Autodesk Inventor part; units mm, degrees
ref_plane "YZ Plane" through (0, 0, 0) normal (1, 0, 0) x (0, 1, 0)
ref_plane "XZ Plane" through (0, 0, 0) normal (0, 1, 0) x (-1, 0, 0)
ref_plane "XY Plane" through (0, 0, 0) normal (0, 0, 1) x (1, 0, 0)
sketch "Skizze1" plane through (0, 0, 0) normal (0, 1, 0) x (-1, 0, 0)
  line L0 (144.9597, 31.6532) -> (-5.0403, 31.6532)
  line L1 (-5.0403, 31.6532) -> (-5.0403, -118.3468)
  line L2 (-5.0403, -118.3468) -> (144.9597, -118.3468)
  line L3 (144.9597, -118.3468) -> (144.9597, 31.6532)
  line L4 (144.9597, 31.6532) -> (-5.0403, -118.3468) construction
  line L5 (-5.0403, 31.6532) -> (144.9597, -118.3468) construction
  point P0 (0, 0)
  point P1 (69.9597, -43.3468)
  dimension "d0" = 150
  dimension "d1" = 150
extrude "Extrusion1" add sketch "Skizze1" along normal blind 5
sketch "Skizze2" plane through (0, 5, 0) normal (0, 1, 0) x (1, 0, 0)
  circle A0 centre (-134.9597, -21.6532) radius 2.5
  circle A1 centre (-134.9597, 108.3468) radius 2.5
  circle A2 centre (-4.9597, -21.6532) radius 2.5
  circle A3 centre (-4.9597, 108.3468) radius 2.5
  line L0 (-144.9597, 118.3468) -> (-144.9597, -31.6532)
  line L1 (-144.9597, -31.6532) -> (5.0403, -31.6532)
  line L2 (5.0403, 118.3468) -> (-144.9597, 118.3468)
  line L3 (5.0403, -31.6532) -> (5.0403, 118.3468)
  point P0 (0, 0)
  dimension "d4" = 5
  dimension "d5" = 5
  dimension "d6" = 5
  dimension "d7" = 5
  dimension "d8" = 10
  dimension "d9" = 10
  dimension "d15" = 10
  dimension "d16" = 10
  dimension "d17" = 10
  dimension "d18" = 10
  dimension "d19" = 10
  dimension "d20" = 10
hole "Bohrung1" at (-134.9597, 5, 21.6532) at (-134.9597, 5, -108.3468) at (-4.9597, 5, -108.3468) at (-4.9597, 5, 21.6532) direction (0, -1, 0) diameter 4.978 depth 19.05 tip angle 118
sketch "Skizze3" plane through (0, 5, 0) normal (0, 1, 0) x (1, 0, 0)
  line L0 (-144.9597, 118.3468) -> (-144.9597, -31.6532)
  line L1 (-144.9597, 18.3468) -> (-124.9597, 18.3468)
  line L2 (-124.9597, 18.3468) -> (-124.9597, 68.3468)
  line L3 (-124.9597, 68.3468) -> (-144.9597, 68.3468)
  line L4 (-144.9597, 68.3468) -> (-144.9597, 18.3468)
  line L5 (-144.9597, -31.6532) -> (5.0403, -31.6532)
  point P0 (0, 0)
  dimension "d28" = 20
  dimension "d29" = 50
  dimension "d30" = 50
extrude "Extrusion2" cut sketch "Skizze3" against normal blind 10
properties part number "Grundplatte1"
Build history of the part. All positions in model axes, mm. A direction names the side the tool comes from. Coordinates: 2 decimals unless noted, no trailing zeros. Write each loop counter-clockwise with the first axis right and the second up, starting at its lowest first coordinate (ties: lowest second). Pieces come first, ordered by that corner, then holes.
(1) 3-axis set-ups, long thin cutter, end or side, ignore diameter. For faces 5 (the cylindrical face through (-5.707, 2.465, 24.027)), 6 (the flat face through (-135, 3, -18.347)): which of +Z, -Z, +X, -X, +Y, -Y reach the whole face in a straight line?
(2) Mould opens along X. For faces 1 (the flat face through (-144.96, 2, 6)), 2 (the cylindrical face through (-137.428, 2.465, 21.329)), 3 (the flat face through (-135, 3, -68.347)), 4 (the cylindrical face through (-137.428, 2.465, -108.671)) say: pulls with the +X half, pulls with the -X half, needs draft (parallel to the pull), parting line crosses it, or undercut.
(3) Pin check, flat tip, straight feed: pin 1 Ø4.5 at (x, z) = (-4.96, 21.65) entering from +Y. Stop position of the tip, or through.
(4) Cut at A-A on z = 22. List the corners of the cut face in (x, y).
(5) Drill centre lines: line 1 (X direction, y = 1.65, z = -59); line 2 (Z direction, x = -138, y = 4.75). Where is each one in solid material? Low to high.
(6) Cut at C-C on z = -42. List the corners of the cut face in (x, y), and give its area (3 significant figures).
(7) Cut at B-B on y = 4.05. List the corners of the cut face in (x, z).
Working result:
1. face 5: +Y, -Y
1. face 6: -X, +Y, -Y
2. face 1: pulls with the -X half
2. face 2: undercut
2. face 3: needs draft
2. face 4: undercut
3. pin 1: passes through
4. outline: (-144.96, 0) - (-137.42, 0) - (-137.42, 5) - (-144.96, 5) - close; (-132.49, 0) - (-7.42, 0) - (-7.42, 5) - (-132.49, 5) - close; (-2.49, 0) - (5.04, 0) - (5.04, 5) - (-2.49, 5) - close
5. line 1: x = -124.96 to 5.04
5. line 2: z = -118.35 to -68.35, -18.35 to 31.65
6. outline: (-124.96, 0) - (5.04, 0) - (5.04, 5) - (-124.96, 5) - close
6. area: 650 mm2
7. outline: (-144.96, -118.35) - (5.04, -118.35) - (5.04, 31.65) - (-144.96, 31.65) - (-144.96, -18.35) - (-124.96, -18.35) - (-124.96, -68.35) - (-144.96, -68.35) - close; hole circle Ø4.98 at (-134.96, -108.35); hole circle Ø4.98 at (-134.96, 21.65); hole circle Ø4.98 at (-4.96, -108.35); hole circle Ø4.98 at (-4.96, 21.65)
